Verification items for the finished model (mm, model axes). Coordinates: 2 decimals unless noted, no trailing zeros. Order: outer loops, then holes, each group sorted by start corner. A loop starts at its lowest first (then second) coordinate and runs counter-clockwise, first axis right, second up.
Q1. Cross-section at D-D, the plane z = 0. Record the boundary of the cut face in (x, y) (3 decimals).
Q2. Thickness scan on line 1 (X direction, y = 2.75, z = 0) (3 decimals); line 2 (Z direction, x = -2.5, y = 2.25); line 3 (X direction, y = 5.25, z = -18). Record the ranges inside material, lowest first.
Q3. Cross-section at A-A, the plane z = -12.5. Record the boundary of the cut face in (x, y).
Q4. Cross-section at C-C, the plane y = 1.75. Record the boundary of the cut face in (x, z) (3 decimals), and give its area (3 significant figures).
Q5. Cross-section at B-B, the plane x = -50.8. Record the boundary of the cut face in (y, z) (3 decimals).
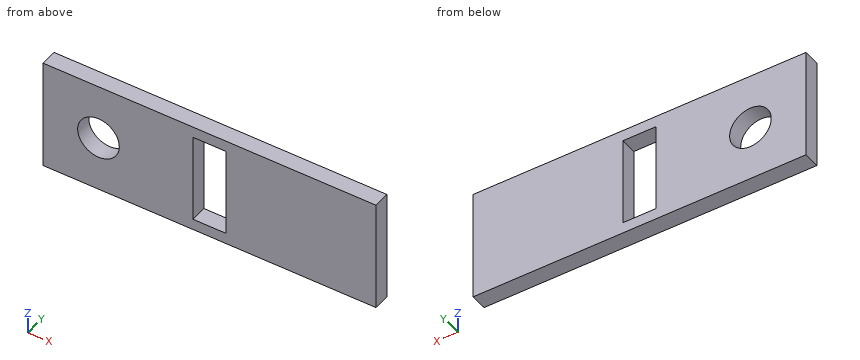
from build123d import *

# Parameters (mm, degrees)
SKETCH1_W           = 152.4
SKETCH1_H           = 50.8
BOSS_EXTRUDE1_DEPTH = 7.62
SKETCH3_R           = 9.525
CUT_EXTRUDE2_DEPTH  = 8.62
SKETCH5_W           = 15.24
SKETCH5_H           = 40.64
CUT_EXTRUDE4_DEPTH  = 8.62


with BuildPart() as part:
    # Sketch1 → Boss-Extrude1 (new body)
    with BuildSketch(Plane(origin=(0, 0, 0), x_dir=(1, 0, 0), z_dir=(0, 1, 0))):
        Rectangle(SKETCH1_W, SKETCH1_H)
    extrude(amount=BOSS_EXTRUDE1_DEPTH)

    # Sketch3 → Cut-Extrude2 (cut, through all)
    with BuildSketch(Plane(origin=(0, 7.62, 0), x_dir=(1, 0, 0), z_dir=(0, 1, 0))):
        with Locations((-50.8, 0)):
            Circle(SKETCH3_R)
    extrude(amount=-CUT_EXTRUDE2_DEPTH, mode=Mode.SUBTRACT)

    # Sketch5 → Cut-Extrude4 (cut, through all)
    with BuildSketch(Plane(origin=(0, 7.62, 0), x_dir=(1, 0, 0), z_dir=(0, 1, 0))):
        Rectangle(SKETCH5_W, SKETCH5_H)
    extrude(amount=-CUT_EXTRUDE4_DEPTH, mode=Mode.SUBTRACT)


solid = part.part
Check values:
1. outline: (-76.2, 0) - (-60.325, 0) - (-60.325, 7.62) - (-76.2, 7.62) - close; (-41.275, 0) - (-7.62, 0) - (-7.62, 7.62) - (-41.275, 7.62) - close; (7.62, 0) - (76.2, 0) - (76.2, 7.62) - (7.62, 7.62) - close
2. line 1: x = -76.2 to -60.325, -41.275 to -7.62, 7.62 to 76.2
2. line 2: z = -25.4 to -20.32, 20.32 to 25.4
2. line 3: x = -76.2 to -7.62, 7.62 to 76.2
3. outline: (-76.2, 0) - (-7.62, 0) - (-7.62, 7.62) - (-76.2, 7.62) - close; (7.62, 0) - (76.2, 0) - (76.2, 7.62) - (7.62, 7.62) - close
4. outline: (-76.2, -25.4) - (76.2, -25.4) - (76.2, 25.4) - (-76.2, 25.4) - close; hole circle Ø19.05 at (-50.8, 0); hole (-7.62, -20.32) - (7.62, -20.32) - (7.62, 20.32) - (-7.62, 20.32) - close
4. area: 6,840 mm2
5. outline: (0, -25.4) - (7.62, -25.4) - (7.62, -9.525) - (0, -9.525) - close; (0, 9.525) - (7.62, 9.525) - (7.62, 25.4) - (0, 25.4) - close
